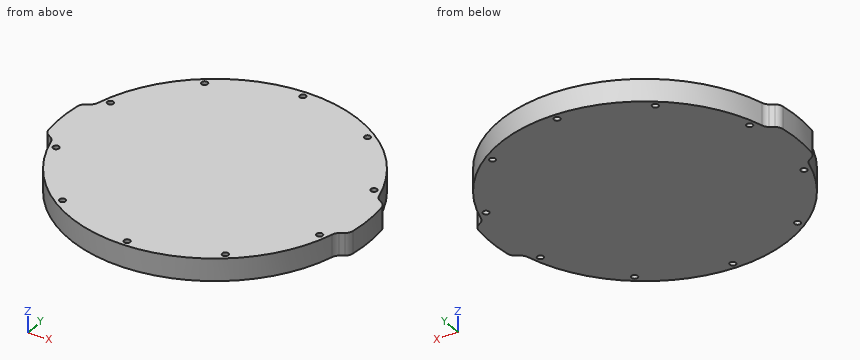
```python
from build123d import *

# Parameters (mm, degrees)
SKETCH1_R           = 1.75
BOSS_EXTRUDE1_DEPTH = 6.35
FILLET1_R           = 5.08


with BuildPart() as part:
    # Sketch1 → Boss-Extrude1 (new, symmetric)
    with BuildSketch(Plane.XY):
        with BuildLine():
            Line((-86.162592811, 15.24), (-80.321852568, 19.05))
            ThreePointArc((-80.321852568, 19.05), (0, 82.55), (80.321852568, 19.05))
            Line((80.321852568, 19.05), (86.162592811, 15.24))
            ThreePointArc((86.162592811, 15.24), (87.5, 0), (86.162592811, -15.24))
            Line((86.162592811, -15.24), (80.321852568, -19.05))
            ThreePointArc((80.321852568, -19.05), (0, -82.55), (-80.321852568, -19.05))
            Line((-80.321852568, -19.05), (-86.162592811, -15.24))
            ThreePointArc((-86.162592811, -15.24), (-87.5, 0), (-86.162592811, 15.24))
        make_face()
        with Locations((0, 78.74)):
            Circle(SKETCH1_R, mode=Mode.SUBTRACT)
        with Locations((46.282210766, 63.701998137)):
            Circle(SKETCH1_R, mode=Mode.SUBTRACT)
        with Locations((74.886190093, 24.331998137)):
            Circle(SKETCH1_R, mode=Mode.SUBTRACT)
        with Locations((74.886190093, -24.331998137)):
            Circle(SKETCH1_R, mode=Mode.SUBTRACT)
        with Locations((46.282210766, -63.701998137)):
            Circle(SKETCH1_R, mode=Mode.SUBTRACT)
        with Locations((0, -78.74)):
            Circle(SKETCH1_R, mode=Mode.SUBTRACT)
        with Locations((-46.282210766, -63.701998137)):
            Circle(SKETCH1_R, mode=Mode.SUBTRACT)
        with Locations((-74.886190093, -24.331998137)):
            Circle(SKETCH1_R, mode=Mode.SUBTRACT)
        with Locations((-74.886190093, 24.331998137)):
            Circle(SKETCH1_R, mode=Mode.SUBTRACT)
        with Locations((-46.282210766, 63.701998137)):
            Circle(SKETCH1_R, mode=Mode.SUBTRACT)
    extrude(amount=BOSS_EXTRUDE1_DEPTH, both=True)

    # Fillet1
    fillet1_edges = [part.edges().sort_by_distance(p)[0] for p in [
        (-86.162592811, -15.24, 0),
        (-86.162592811, 15.24, 0),
        (-80.321852568, 19.05, 0),
        (80.321852568, 19.05, 0),
        (86.162592811, 15.24, 0),
        (86.162592811, -15.24, 0),
        (80.321852568, -19.05, 0),
        (-80.321852568, -19.05, 0),
    ]]
    fillet(fillet1_edges, radius=FILLET1_R)


solid = part.part
```
Geometry check sheet. Reference: the model listing, model coordinates, mm. Round coordinates to 2 decimals unless told otherwise and drop trailing zeros. Loops run counter-clockwise (first coordinate to the right, second up) from the corner with the lowest first, then second, coordinate; pieces in that order, holes last. Notation, with made-up numbers: (23, 58) - (53, 58) arc R34 cw to (53, 88) - close; hole circle Ø10 at (43.25, 79.5). An arc over 180 degrees is marked (long way). Write each question's results on one line, items separated by ' | '. Start each with the question number.
Q1. Cross-section at A-A on z = 2.5. State how many separate pieces and enclosed holes the cut face has, and give its area (3 significant figures).
Q2. Gauge pin test, flat ends, axial feed: P1, Ø3, axis at x = 74.89, y = 24.33, coming from the +Z side; P2, Ø6, axis at x = -37, z = -2, coming from the -Y side; P3, Ø6, axis at y = -43, z = -0.5, coming from the -X side; P4, Ø1.5, axis at x = 65, z = 4, coming from the -Y side. Record the tip position at first contact, or that the pin passes through.
Q3. Thickness scan on line 1 (Y direction, x = 74.5, z = -3.75); line 2 (X direction, y = -24, z = 2.25); line 3 (X direction, y = -2, z = -0.25). Record the ranges inside material, lowest first. Write a range as [from, to].
Q4. Cross-section at C-C on x = -29.5. Enter the section's corners in (y, z), and give its area (3 significant figures).
Q5. Cross-section at B-B on y = 55. Enter the section's corners in (x, z).
Answers below:
1) separate pieces: 1 | enclosed holes: 10 | area: 21,700 mm²
2) P1: passes through | P2: stops at y = -75.22 | P3: stops at x = -72.21 | P4: stops at y = -51.83
3) line 1: y = [-35.56, -26.04], [-22.63, 22.63], [26.04, 35.56] | line 2: x = [-78.98, -76.6], [-73.17, 73.17], [76.6, 78.98] | line 3: x = [-87.48, 87.48]
4) outline: (-77.1, -6.35) - (77.1, -6.35) - (77.1, 6.35) - (-77.1, 6.35) - close | area: 1,960 mm²
5) outline: (-61.56, -6.35) - (61.56, -6.35) - (61.56, 6.35) - (-61.56, 6.35) - close
